Part print with two shaded views. Sizes in mm from the minimum x, y, z corner. Coordinates: 2 decimals unless noted, no trailing zeros. Loops run counter-clockwise (first coordinate to the right, second up) from the corner with the lowest first, then second, coordinate; pieces in that order, holes last.
Item 1: Drill centre lines: line 1 along X through (y, z) = (21.5, 6); line 2 along X through (y, z) = (75.5, 6); line 3 along X through (y, z) = (356, 9.25). Where is each one in solid material? Low to high.
Item 2: Cut at C-C (y = 136.5). List the corners of the cut face in (x, z).
Item 3: Cut at A-A (y = 63.5). List the corners of the cut face in (x, z).
Item 4: Cut at B-B (z = 7.5). List the corners of the cut face in (x, y) (3 decimals), and give its area (3 significant figures).
Item 5: Flat gauge pins, fed straight in: pin 1 (4 mm diameter, centred on y = 324.5, z = 7, fed in from +X); pin 2 (5 mm diameter, centred on y = 260, z = 8, fed in from -X); pin 3 (10 mm diameter, centred on x = 119, y = 113.5, fed in from -Z); pin 4 (6.5 mm diameter, centred on x = 9.5, z = 4.5, fed in from -Y). Where does each tip first touch, or does it go through?
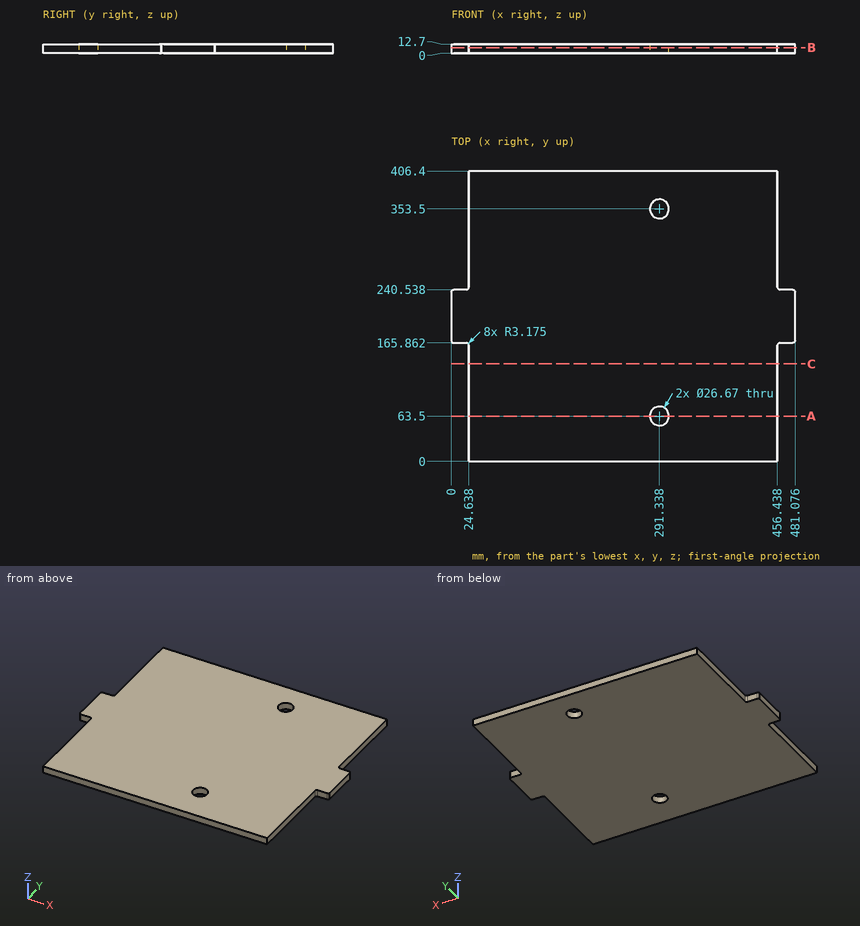
Filled sheet:
1. line 1: x = 24.64 to 456.44
1. line 2: x = 24.64 to 285.52, 297.15 to 456.44
1. line 3: x = 24.64 to 278.24, 304.44 to 456.44
2. outline: (24.64, 0) - (456.44, 0) - (456.44, 12.7) - (24.64, 12.7) - close
3. outline: (24.64, 0) - (278, 0) - (278, 12.7) - (24.64, 12.7) - close; (304.67, 0) - (456.44, 0) - (456.44, 12.7) - (304.67, 12.7) - close
4. outline: (0, 169.037) arc R3.175 ccw to (3.175, 165.862) - (21.463, 165.862) arc R3.175 cw to (24.638, 162.687) - (24.638, 0) - (456.438, 0) - (456.438, 162.687) arc R3.175 cw to (459.613, 165.862) - (477.901, 165.862) arc R3.175 ccw to (481.076, 169.037) - (481.076, 237.363) arc R3.175 ccw to (477.901, 240.538) - (459.613, 240.538) arc R3.175 cw to (456.438, 243.713) - (456.438, 406.4) - (24.638, 406.4) - (24.638, 243.713) arc R3.175 cw to (21.463, 240.538) - (3.175, 240.538) arc R3.175 ccw to (0, 237.363) - close; hole circle Ø26.67 at (291.338, 63.5); hole circle Ø26.67 at (291.338, 353.5)
4. area: 178,000 mm2
5. pin 1: stops at x = 456.44
5. pin 2: stops at x = 24.64
5. pin 3: stops at z = 0
5. pin 4: stops at y = 165.86
